from build123d import *

# Parameters (mm, degrees)
FILLET_1_R    = 2
SCALE_1_SCALE = 0.338461538
SCALE_2_SCALE = 0.5


with BuildPart() as part:
    # 草图1 → 旋转1 (revolve)
    with BuildSketch(Plane.XY, mode=Mode.PRIVATE) as revolve_1_sk:
        with BuildLine():
            Line((-15.5, 53), (-8.94427191, 53))
            ThreePointArc((-8.94427191, 53), (0, 57), (8.94427191, 53))
            Line((8.94427191, 53), (15.5, 53))
            Line((15.5, 53), (15.5, 65))
            Line((15.5, 65), (-15.5, 65))
            Line((-15.5, 65), (-15.5, 53))
        make_face()
    revolve(revolve_1_sk.sketch.rotate(Axis((0, 0, 0), (1, 0, 0)), 90), axis=Axis((0, 0, 0), (1, 0, 0)))

    # 圆角1
    fillet_1_edges = [part.edges().sort_by_distance(p)[0] for p in [
        (15.5, 0, -65),
        (-15.5, 0, -65),
    ]]
    fillet(fillet_1_edges, radius=FILLET_1_R)


with BuildPart() as part_1:
    # 缩放比例1: scaled about (0, 0, 0)
    add(part.part.scale(SCALE_1_SCALE))


with BuildPart() as part_2:
    # 缩放比例2: scaled about (0, 0, 0)
    add(part_1.part.scale(SCALE_2_SCALE))


solid = part_2.part
Can you work these out from the model? Positions are in its coordinate system, mm. Round coordinates to 2 decimals unless told otherwise and drop trailing zeros. Write each loop counter-clockwise with the first axis right and the second up, starting at its lowest first coordinate (ties: lowest second). Pieces come first, ordered by that corner, then holes. Notation, with made-up numbers: (88.25, -38) - (95.25, -38) arc R24 ccw to (95.25, -6) - close; hole circle Ø10 at (4, 74). An arc over 180 degrees is marked (long way). Write each question's results on one line, items separated by ' | '. Start each with the question number.
1) For pin 1 Ø3 at (x, z) = (1.5, -2) entering from -Y; pin 2 Ø2 at (y, z) = (-6, 4) entering from -X; pin 3 Ø1 at (x, y) = (-0.5, -8) entering from +Z; pin 4 Ø4 at (y, z) = (-1, -7) entering from +X, each with a flat end and sliding along its axis, tell me the tip position at first contact or that it passes through.
2) Suppose I cut it at A-A (z = 0). List the corners of the cut face in (x, y) for me, and give its area (3 significant figures).
3) We'd pull the mould along Z, two halves only. Please class faces 1 (the cylindrical face through (-2.061, -2.694, 8.555)), 2 (the cylindrical face through (-0.032, 9.759, 5.076)), 3 (the flat face through (2.623, -9, 2)): released by +Z, released by -Z, zero draft, split by the parting line, or undercut.
4) Please list where these lines run through material, in increasing order: line 1 (Y direction, x = -2, z = 0); line 2 (Y direction, x = 1.8, z = -4); line 3 (Z direction, x = -0.8, y = -3).
Here are the results:
1) pin 1: stops at y = -10.99 | pin 2: passes through | pin 3: stops at z = 8.05 | pin 4: stops at x = 2.62
2) outline: (-2.62, -10.66) arc R0.34 ccw to (-2.28, -11) - (2.28, -11) arc R0.34 ccw to (2.62, -10.66) - (2.62, -8.97) - (1.51, -8.97) arc R2.03 cw to (-1.51, -8.97) - (-2.62, -8.97) - close; (-2.62, 8.97) - (-1.51, 8.97) arc R2.03 cw to (1.51, 8.97) - (2.62, 8.97) - (2.62, 10.66) arc R0.34 ccw to (2.28, 11) - (-2.28, 11) arc R0.34 ccw to (-2.62, 10.66) - close | area: 18.4 mm2
3) face 1: undercut | face 2: split by the parting line | face 3: zero draft
4) line 1: y = -11 to -8.97, 8.97 to 11 | line 2: y = -10.25 to -8.03, 8.03 to 10.25 | line 3: z = -10.58 to -8.99, 8.99 to 10.58
